Verification items for the finished model (mm, model axes). Give positions to 0.01 mm unless a question says otherwise; leave off trailing zeros. Write each loop counter-clockwise with the first axis right and the second up, starting at its lowest first coordinate (ties: lowest second). Pieces come first, ordered by that corner, then holes.
Autodesk Inventor part; units mm, degrees
ref_plane "mss_or_XY" through (0, 0, 0) normal (1, 0, 0) x (0, 0, -1)
ref_plane "mss_or_YZ" through (0, 0, 0) normal (0, 0, -1) x (0, 1, 0)
ref_plane "mss_or_ZX" through (0, 0, 0) normal (0, 1, 0) x (1, 0, 0)
sketch "Sketch_1" plane through (0, 0, 0) normal (0, 0, 1) x (1, 0, 0)
  line L0 (2, 0) -> (0, 0)
  line L1 (0, 2.92) -> (0, 2.52)
  line L2 (0, 2.52) -> (0.6475, 2.52)
  arc A0 (1.3525, 2.52) -> (0.6475, 2.52) centre (1, 2.25) ccw
  line L3 (1.3525, 2.52) -> (2, 2.52)
  line L4 (2, 2.52) -> (2, 2.92)
  arc A1 (2, 2.92) -> (1.92, 3) centre (1.92, 2.92) ccw
  line L5 (1.92, 3) -> (0.08, 3)
  arc A2 (0.08, 3) -> (0, 2.92) centre (0.08, 2.92) ccw
revolve "Revolution1" add sketch "Sketch_1" angle 360 about axis through (2, 0, 0) along (1, 0, 0)
ref_plane "mss_or_XY" through (0, 0, 0) normal (1, 0, 0) x (0, 0, -1)
ref_plane "mss_or_YZ" through (0, 0, 0) normal (0, 0, -1) x (0, 1, 0)
ref_plane "mss_or_ZX" through (0, 0, 0) normal (0, 1, 0) x (1, 0, 0)
ref_plane "mss_or11_XY" through (2.5, 0, 0) normal (1, 0, 0) x (0, 0, -1)
ref_plane "mss_or11_YZ" through (2.5, 0, 0) normal (0, 0, -1) x (0, 1, 0)
ref_plane "mss_or11_ZX" through (2.5, 0, 0) normal (0, 1, 0) x (1, 0, 0)
ref_plane "mss_or2_1_XY" through (1, 2.25, 0) normal (1, 0, 0) x (0, 0, -1)
ref_plane "mss_or2_1_YZ" through (1, 2.25, 0) normal (0, 0, -1) x (0, 1, 0)
ref_plane "mss_or2_1_ZX" through (1, 2.25, 0) normal (0, 1, 0) x (1, 0, 0)
ref_plane "mss_or2_2_XY" through (1, 1.7236, 1.4463) normal (1, 0, 0) x (0, 0, -1)
ref_plane "mss_or2_2_YZ" through (1, 1.7236, 1.4463) normal (0, 0, -1) x (0, 1, 0)
ref_plane "mss_or2_2_ZX" through (1, 1.7236, 1.4463) normal (0, 1, 0) x (1, 0, 0)
ref_plane "mss_or2_3_XY" through (1, 0.3907, 2.2158) normal (1, 0, 0) x (0, 0, -1)
ref_plane "mss_or2_3_YZ" through (1, 0.3907, 2.2158) normal (0, 0, -1) x (0, 1, 0)
ref_plane "mss_or2_3_ZX" through (1, 0.3907, 2.2158) normal (0, 1, 0) x (1, 0, 0)
ref_plane "mss_or2_4_XY" through (1, -1.125, 1.9486) normal (1, 0, 0) x (0, 0, -1)
ref_plane "mss_or2_4_YZ" through (1, -1.125, 1.9486) normal (0, 0, -1) x (0, 1, 0)
ref_plane "mss_or2_4_ZX" through (1, -1.125, 1.9486) normal (0, 1, 0) x (1, 0, 0)
ref_plane "mss_or2_5_XY" through (1, -2.1143, 0.7695) normal (1, 0, 0) x (0, 0, -1)
ref_plane "mss_or2_5_YZ" through (1, -2.1143, 0.7695) normal (0, 0, -1) x (0, 1, 0)
ref_plane "mss_or2_5_ZX" through (1, -2.1143, 0.7695) normal (0, 1, 0) x (1, 0, 0)
ref_plane "mss_or2_6_XY" through (1, -2.1143, -0.7695) normal (1, 0, 0) x (0, 0, -1)
ref_plane "mss_or2_6_YZ" through (1, -2.1143, -0.7695) normal (0, 0, -1) x (0, 1, 0)
ref_plane "mss_or2_6_ZX" through (1, -2.1143, -0.7695) normal (0, 1, 0) x (1, 0, 0)
ref_plane "mss_or2_7_XY" through (1, -1.125, -1.9486) normal (1, 0, 0) x (0, 0, -1)
ref_plane "mss_or2_7_YZ" through (1, -1.125, -1.9486) normal (0, 0, -1) x (0, 1, 0)
ref_plane "mss_or2_7_ZX" through (1, -1.125, -1.9486) normal (0, 1, 0) x (1, 0, 0)
ref_plane "mss_or2_8_XY" through (1, 0.3907, -2.2158) normal (1, 0, 0) x (0, 0, -1)
ref_plane "mss_or2_8_YZ" through (1, 0.3907, -2.2158) normal (0, 0, -1) x (0, 1, 0)
ref_plane "mss_or2_8_ZX" through (1, 0.3907, -2.2158) normal (0, 1, 0) x (1, 0, 0)
ref_plane "mss_or2_9_XY" through (1, 1.7236, -1.4463) normal (1, 0, 0) x (0, 0, -1)
ref_plane "mss_or2_9_YZ" through (1, 1.7236, -1.4463) normal (0, 0, -1) x (0, 1, 0)
ref_plane "mss_or2_9_ZX" through (1, 1.7236, -1.4463) normal (0, 1, 0) x (1, 0, 0)
ref_plane "mss_or21_1_XY" through (1.25, 2.25, 0) normal (1, 0, 0) x (0, 0, -1)
ref_plane "mss_or21_1_YZ" through (1.25, 2.25, 0) normal (0, 0, -1) x (0, 1, 0)
ref_plane "mss_or21_1_ZX" through (1.25, 2.25, 0) normal (0, 1, 0) x (1, 0, 0)
ref_plane "mss_or21_2_XY" through (1.25, 1.7236, 1.4463) normal (1, 0, 0) x (0, 0, -1)
ref_plane "mss_or21_2_YZ" through (1.25, 1.7236, 1.4463) normal (0, 0, -1) x (0, 1, 0)
ref_plane "mss_or21_2_ZX" through (1.25, 1.7236, 1.4463) normal (0, 1, 0) x (1, 0, 0)
ref_plane "mss_or21_3_XY" through (1.25, 0.3907, 2.2158) normal (1, 0, 0) x (0, 0, -1)
ref_plane "mss_or21_3_YZ" through (1.25, 0.3907, 2.2158) normal (0, 0, -1) x (0, 1, 0)
ref_plane "mss_or21_3_ZX" through (1.25, 0.3907, 2.2158) normal (0, 1, 0) x (1, 0, 0)
ref_plane "mss_or21_4_XY" through (1.25, -1.125, 1.9486) normal (1, 0, 0) x (0, 0, -1)
ref_plane "mss_or21_4_YZ" through (1.25, -1.125, 1.9486) normal (0, 0, -1) x (0, 1, 0)
ref_plane "mss_or21_4_ZX" through (1.25, -1.125, 1.9486) normal (0, 1, 0) x (1, 0, 0)
ref_plane "mss_or21_5_XY" through (1.25, -2.1143, 0.7695) normal (1, 0, 0) x (0, 0, -1)
ref_plane "mss_or21_5_YZ" through (1.25, -2.1143, 0.7695) normal (0, 0, -1) x (0, 1, 0)
ref_plane "mss_or21_5_ZX" through (1.25, -2.1143, 0.7695) normal (0, 1, 0) x (1, 0, 0)
ref_plane "mss_or21_6_XY" through (1.25, -2.1143, -0.7695) normal (1, 0, 0) x (0, 0, -1)
ref_plane "mss_or21_6_YZ" through (1.25, -2.1143, -0.7695) normal (0, 0, -1) x (0, 1, 0)
ref_plane "mss_or21_6_ZX" through (1.25, -2.1143, -0.7695) normal (0, 1, 0) x (1, 0, 0)
ref_plane "mss_or21_7_XY" through (1.25, -1.125, -1.9486) normal (1, 0, 0) x (0, 0, -1)
ref_plane "mss_or21_7_YZ" through (1.25, -1.125, -1.9486) normal (0, 0, -1) x (0, 1, 0)
ref_plane "mss_or21_7_ZX" through (1.25, -1.125, -1.9486) normal (0, 1, 0) x (1, 0, 0)
ref_plane "mss_or21_8_XY" through (1.25, 0.3907, -2.2158) normal (1, 0, 0) x (0, 0, -1)
ref_plane "mss_or21_8_YZ" through (1.25, 0.3907, -2.2158) normal (0, 0, -1) x (0, 1, 0)
ref_plane "mss_or21_8_ZX" through (1.25, 0.3907, -2.2158) normal (0, 1, 0) x (1, 0, 0)
ref_plane "mss_or21_9_XY" through (1.25, 1.7236, -1.4463) normal (1, 0, 0) x (0, 0, -1)
ref_plane "mss_or21_9_YZ" through (1.25, 1.7236, -1.4463) normal (0, 0, -1) x (0, 1, 0)
ref_plane "mss_or21_9_ZX" through (1.25, 1.7236, -1.4463) normal (0, 1, 0) x (1, 0, 0)
properties part number "673 Outer ring"
Item 1: Scan lines: line 1 along Z through (x, y) = (1.75, 0); line 2 along Y through (x, z) = (0.9, 1.4); line 3 along Y through (x, z) = (1.2, 0.2). Record each from-to range of solid material in increasing order.
Answer key:
line 1: z = -3 to -2.52, 2.52 to 3
line 2: y = -2.65 to -2.29, 2.29 to 2.65
line 3: y = -2.99 to -2.64, 2.64 to 2.99
Item 2: Depth check by flat-ended pin: pin 1 (3 mm diameter, centred on y = 0, z = 0, fed in from -X). Enter the tip coordinate at first touch or a pass-through.
Answer key:
pin 1: passes through
Item 3: Sectioned sample at A-A on z = 0. Record the cut outline in (x, y).
Answer key:
outline: (0, -2.92) arc R0.08 ccw to (0.08, -3) - (1.92, -3) arc R0.08 ccw to (2, -2.92) - (2, -2.52) - (1.35, -2.52) arc R0.44 cw to (0.65, -2.52) - (0, -2.52) - close; (0, 2.52) - (0.65, 2.52) arc R0.44 cw to (1.35, 2.52) - (2, 2.52) - (2, 2.92) arc R0.08 ccw to (1.92, 3) - (0.08, 3) arc R0.08 ccw to (0, 2.92) - close
Item 4: Sectioned sample at D-D on x = 0.85. Record the cut outline in (y, z).
Answer key:
outline: circle Ø6 at (0, 0); hole circle Ø5.34 at (0, 0)
Item 5: Sectioned sample at C-C on x = 0.35. Record the cut outline in (y, z), then the cut area to 3 significant figures.
Answer key:
outline: circle Ø6 at (0, 0); hole circle Ø5.04 at (0, 0)
area: 8.32 mm2
Item 6: Release check for a two-part mould opening along Y. For faces 1 (the face through (1, -3, 0)), 2 (the face through (0.33, -2, -1.53)) record: released by +Y, released by -Y, zero draft, split by the parting line, or undercut.
Answer key:
face 1: split by the parting line
face 2: undercut
